CAD build for the part. Positions are in the model's coordinates, mm. A direction names the side the tool comes from. Round coordinates to 2 decimals unless told otherwise and drop trailing zeros. Write each loop counter-clockwise with the first axis right and the second up, starting at its lowest first coordinate (ties: lowest second). Pieces come first, ordered by that corner, then holes. Notation, with made-up numbers: (37.25, -39.75) - (51.25, -39.75) arc R17 ccw to (51.25, -13.75) - close; hole circle Ø1 at (14.25, 75). An arc over 180 degrees is marked (long way). Answer in a Markdown table with one row per item.
```python
from build123d import *


with BuildPart() as cono001:
    # Cone001 → Cone001 (revolve)
    with BuildSketch(Plane(origin=(0, 0, 2.5), x_dir=(1, 0, 0), z_dir=(0, -1, 0))):
        Polygon((0, 0), (195, 0), (395, 397.5), (0, 397.5), align=None)
    revolve(axis=Axis((0, 0, 2.5), (0, 0, 1)))


with BuildPart() as cut:
    # Cone → Cone (revolve)
    with BuildSketch(Plane.XZ):
        Polygon((0, 0), (200, 0), (400, 400), (0, 400), align=None)
    revolve(axis=Axis((0, 0, 0), (0, 0, 1)))

    # Cut: cut Cono001
    add(cono001.part, mode=Mode.SUBTRACT)


solid = cut.part
```
Q1. Pull direction X, two halves, no side cores. Call faces 3 (the conical face through (-186.28, -142.83, 69.47)), 4 (the conical face through (219.12, 69.01, 71.53)), 5 (the flat face through (294, -265, 400)): released by +X, released by -X, zero draft, split by the parting line, or undercut.
Computed:
| item | result |
|---|---|
| face 3 | split by the parting line |
| face 4 | undercut |
| face 5 | zero draft |
Q2. Drill centre lines: line 1 (X direction, y = -114, z = 260); line 2 (Z direction, x = 7, y = -89); line 3 (X direction, y = -108.5, z = 314). Where is each one in solid material? Low to high.
Computed:
| item | result |
|---|---|
| line 1 | x = -309.68 to -303.88, 303.88 to 309.68 |
| line 2 | z = 0 to 2.5 |
| line 3 | x = -340.11 to -334.58, 334.58 to 340.11 |
Q3. Saw through at A-A on x = 0. List the corners of the cut face in (y, z).
Computed:
| item | result |
|---|---|
| outline | (-400, 400) - (-200, 0) - (200, 0) - (400, 400) - (395, 400) - (195, 2.5) - (-195, 2.5) - (-395, 400) - close |
Q4. 3-axis set-ups, long thin cutter, end or side, ignore diameter. For faces 1 (the flat face through (3, 3, 0)), 2 (the flat face through (3, 3, 2.5)): which of +Z, -Z, +X, -X, +Y, -Y reach the whole face in a straight line?
Computed:
| item | result |
|---|---|
| face 1 | -Z, +X, -X, +Y, -Y |
| face 2 | +Z |
Q5. Saw through at C-C on z = 182. List the corners of the cut face in (x, y).
Computed:
| item | result |
|---|---|
| outline | circle Ø582 at (0, 0); hole circle Ø570.63 at (0, 0) |
Q6. Flat gauge pins, fed straight in: pin 1 (5 mm diameter, centred on y = -147, z = 230, fed in from +X); pin 2 (6 mm diameter, centred on y = 232.5, z = 260.5, fed in from -X); pin 3 (6 mm diameter, centred on y = -306.5, z = 304.5, fed in from -X). Where does each tip first touch, or does it go through?
Computed:
| item | result |
|---|---|
| pin 1 | stops at x = 280.52 |
| pin 2 | stops at x = -238.15 |
| pin 3 | stops at x = -179.59 |
Q7. Saw through at D-D on z = 263.5. List the corners of the cut face in (x, y), then the cut area to 3 significant figures.
Computed:
| item | result |
|---|---|
| outline | circle Ø663.5 at (0, 0); hole circle Ø652.64 at (0, 0) |
| area | 11,200 mm2 |
